Autodesk Fusion 360 part; units mm, degrees
sketch "front" plane through (0, 0, 0) normal (0, 1, 0) x (1, 0, 0) in component "LM8UU"
  circle A0 centre (0, 0) radius 4
  circle A1 centre (0, 0) radius 7
  circle A2 centre (0, 0) radius 7.5
  circle A3 centre (0, 0) radius 4.1
  dimension "d1" = 8
  dimension "d2" = 14
  dimension "d3" = 15
  dimension "d20" = 8.2
extrude "Extrude1" add sketch "front" along normal blind 3.25 contours A1 | A2 | A3 in component "LM8UU"
extrude "Extrude2" add sketch "front" along normal blind 1.1 from surface at 3.25 contours A1 | A3 in component "LM8UU"
extrude "Extrude3" add sketch "front" along normal blind 15.3 from surface at 4.35 contours A1 | A2 | A3 in component "LM8UU"
extrude "Extrude4" add sketch "front" along normal blind 1.1 from surface at 19.65 contours A1 | A3 in component "LM8UU"
extrude "Extrude5" add sketch "front" along normal blind 3.25 from surface at 20.75 contours A1 | A2 | A3 in component "LM8UU"
fillet "Fillet1" radius 0.25 2 edges at (-6.9925, 0, 2.7121) (-6.9925, 24, 2.7121) in component "LM8UU"
extrude "Extrude6" cut sketch "front" along normal blind 0.01 contours A1 in component "LM8UU"
extrude "Extrude7" cut sketch "front" along normal blind 0.01 from surface at 23.99 contours A1 in component "LM8UU"
component "LM8UU" placed x (1, 0, 0) y (0, 1, 0) z (0, 0, 1) at (0, 0, 0)
equation "d9 = 3.25 mm + 1.1 mm"
equation "d10 = 17.5 mm - 2.2 mm"
equation "d12 = 3.25 mm + 17.5 mm - 1.1 mm"
equation "d15 = 3.25 mm + 17.5 mm"
equation "d23 = 24 mm - 0.01 mm"
Work out the finished part from the listing and answer in its coordinate system (mm). A direction names the side the tool comes from. Coordinates: 2 decimals unless noted, no trailing zeros. Loops run counter-clockwise (first coordinate to the right, second up) from the corner with the lowest first, then second, coordinate; pieces in that order, holes last. Notation, with made-up numbers: M 50,7.5 L 89,7.5 A20 ccw 89,15.5 Z; hole C -38.75,84.25 d7. An arc over 180 degrees is marked long. Answer in a Markdown table with one row per item. Add a question column.
1. A tool of negligible diameter and unlimited length cuts with its end or side. For faces 4 (the flat face through (7, 19.65, -2)), 5 (the cylindrical face through (-7.493, 1.729, 0.33)), from which of +Z, -Z, +X, -X, +Y, -Y can it reach the whole face along a straight path? Write none if from no direction.
2. Find section A-A, the plane y = 18.5. Write down the section's boundary in (x, z), then the cut area to 3 significant figures.
3. Flat-ended cylindrical pins translate along their axes: P1, Ø5, axis at y = 5, z = -4, coming from the +X side; P2, Ø4, axis at y = 18, z = 3, coming from the +X side. Find the tip coordinate at first contact, or state that the pin passes through.
4. The mould has two halves that part along Z. Classify faces 1 (the cylindrical face through (-7.493, 11.893, 0.33)), 2 (the cylindrical face through (-0.867, 11.832, -3.905)), 3 (the flat face through (7, 20.75, -2)): pulls with the +Z half, pulls with the -Z half, needs draft (parallel to the pull), parting line crosses it, or undercut.
5. Consider L1, parallel to Y at x = -5.75, z = -4.25; L2, parallel to X at y = 16.75, z = 0; L3, parallel to Y at x = 3.5, z = 5. Determine where each line is inside the solid, lowest interval first.
Reported:
| question | item | result |
|---|---|---|
| 1 | face 4 | none |
| 1 | face 5 | +Y, -Y |
| 2 | outline | C 0,0 d15; hole C 0,0 d8 |
| 2 | area | 126 mm^2 |
| 3 | P1 | stops at x = 7.35 |
| 3 | P2 | stops at x = 7.43 |
| 4 | face 1 | parting line crosses it |
| 4 | face 2 | undercut |
| 4 | face 3 | needs draft |
| 5 | L1 | y = 0 to 3.25, 4.35 to 19.65, 20.75 to 24 |
| 5 | L2 | x = -7.5 to -4, 4 to 7.5 |
| 5 | L3 | y = 0.01 to 23.99 |
